from build123d import *

# Parameters (mm, degrees)
ESQUISSE1_W                   = 105
ESQUISSE1_H                   = 105
ESQUISSE1_W_2                 = 85
ESQUISSE1_H_2                 = 85
BOSS_EXTRU_3_DEPTH            = 88
BOSS_EXTRU_4_DEPTH            = 105
ESQUISSE7_W                   = 40
ESQUISSE7_H                   = 40
ESQUISSE7_W_2                 = 20
ESQUISSE7_H_2                 = 20
BOSS_EXTRU_11_DEPTH           = 110.5
ENL_V_MAT_EXTRU_9_REACH       = 242.562
ESQUISSE13_W                  = 10
ESQUISSE13_H                  = 20
BOSS_EXTRU_12_DEPTH           = 2.5
ESQUISSE17_R                  = 5
ESQUISSE17_W                  = 40
ESQUISSE17_H                  = 20
BOSS_EXTRU_13_DEPTH           = 52.5
ENL_V_MAT_EXTRU_12_DEPTH      = 265.326910813
ENL_V_MAT_EXTRU_12_DEPTH_BACK = 265.326910813
ESQUISSE18_R                  = 5
ENL_V_MAT_EXTRU_13_REACH      = 236.819
ESQUISSE19_W                  = 10
ESQUISSE19_H                  = 20
CONG_1_R                      = 10
ENL_V_MAT_EXTRU_15_DEPTH      = 88


with BuildPart() as part:
    # Esquisse1 → Boss.-Extru.3 (new body)
    with BuildSketch(Plane(origin=(0, 0, 0), x_dir=(1, 0, 0), z_dir=(0, 1, 0))):
        Rectangle(ESQUISSE1_W, ESQUISSE1_H)
        Rectangle(ESQUISSE1_W_2, ESQUISSE1_H_2, mode=Mode.SUBTRACT)
    extrude(amount=BOSS_EXTRU_3_DEPTH)

    # Esquisse3 → Boss.-Extru.4 (add)
    with BuildSketch(Plane.XY.offset(52.5)):
        Polygon((52.5, 6), (52.5, 0), (96.658434537, 0), (130.222419784, 40), (190.222419784, 40), (190.222419784, 46), (127.424573836, 46), (93.860588588, 6), align=None)
    extrude(amount=-BOSS_EXTRU_4_DEPTH)

    # Esquisse7 → Boss.-Extru.11 (add)
    with BuildSketch(Plane.XZ.offset(-40)):
        with Locations((190.222419784, 0)):
            Rectangle(ESQUISSE7_W, ESQUISSE7_H)
        with Locations((190.222419784, 0)):
            Rectangle(ESQUISSE7_W_2, ESQUISSE7_H_2, mode=Mode.SUBTRACT)
    extrude(amount=-BOSS_EXTRU_11_DEPTH)

    # Esquisse13 → Enlèv. mat.-Extru.9 (cut, up to next)
    with BuildSketch(Plane(origin=(0, 46, 0), x_dir=(1, 0, 0), z_dir=(0, 1, 0)), mode=Mode.PRIVATE) as enl_v_mat_extru_9_sk1:
        with Locations((185.222419784, 0)):
            Rectangle(ESQUISSE13_W, ESQUISSE13_H)
    enl_v_mat_extru_9_tool1 = extrude(enl_v_mat_extru_9_sk1.sketch, amount=-ENL_V_MAT_EXTRU_9_REACH, mode=Mode.PRIVATE) & part.part
    add(enl_v_mat_extru_9_tool1.solids().sort_by_distance((185.22242, 46, 0))[0], mode=Mode.SUBTRACT)

    # Esquisse14 → Boss.-Extru.12 (add, symmetric)
    with BuildSketch(Plane.XY):
        Polygon((52.5, 88), (101.965319391, 88), (154.40904634, 150.5), (170.222419784, 150.5), (170.222419784, 46), (127.424573836, 46), (93.860588588, 6), (52.5, 6), align=None)
    extrude(amount=BOSS_EXTRU_12_DEPTH, both=True)

    # Esquisse17 → Boss.-Extru.13 (add, symmetric)
    # profile 1 of 2: a face of its own
    with BuildSketch(Plane.XY):
        Polygon((44, 20), (44, 0), (77.5, 0), (77.5, 6), (77.5, 20), align=None)
        with Locations((67.5, 10)):
            Circle(ESQUISSE17_R, mode=Mode.SUBTRACT)
    # profile 2 of 2: a face of its own
    with BuildSketch(Plane.XY):
        with Locations((170.222419784, 50)):
            Rectangle(ESQUISSE17_W, ESQUISSE17_H)
        with Locations((160.222419784, 50)):
            Circle(ESQUISSE17_R, mode=Mode.SUBTRACT)
    extrude(amount=BOSS_EXTRU_13_DEPTH, both=True)

    # Esquisse18 → Enlèv. mat.-Extru.12 (cut, two sides: drawn at the far end of the back side and taken through both)
    with BuildSketch(Plane.XY.offset(2.5).offset(-ENL_V_MAT_EXTRU_12_DEPTH_BACK)):
        with Locations((160.222419784, 50)):
            Circle(ESQUISSE18_R)
        with Locations((67.5, 10)):
            Circle(ESQUISSE18_R)
    extrude(amount=ENL_V_MAT_EXTRU_12_DEPTH + ENL_V_MAT_EXTRU_12_DEPTH_BACK, mode=Mode.SUBTRACT)

    # Esquisse19 → Enlèv. mat.-Extru.13 (cut, up to next)
    with BuildSketch(Plane(origin=(0, 60, 0), x_dir=(1, 0, 0), z_dir=(0, 1, 0)), mode=Mode.PRIVATE) as enl_v_mat_extru_13_sk1:
        with Locations((185.222419784, 0)):
            Rectangle(ESQUISSE19_W, ESQUISSE19_H)
    enl_v_mat_extru_13_tool1 = extrude(enl_v_mat_extru_13_sk1.sketch, amount=-ENL_V_MAT_EXTRU_13_REACH, mode=Mode.PRIVATE) & part.part
    add(enl_v_mat_extru_13_tool1.solids().sort_by_distance((185.22242, 60, 0))[0], mode=Mode.SUBTRACT)

    # Congé1
    cong_1_edges = [part.edges().sort_by_distance(p)[0] for p in [
        (93.860588588, 6, 27.5),
        (127.424573836, 46, 27.5),
        (154.40904634, 150.5, 0),
        (101.965319391, 88, 0),
        (77.5, 20, 27.5),
        (77.5, 20, -27.5),
        (150.222419784, 60, 27.5),
        (150.222419784, 60, -27.5),
        (127.424573836, 46, -27.5),
        (93.860588588, 6, -27.5),
        (96.658434537, 0, 0),
        (130.222419784, 40, 0),
    ]]
    fillet(cong_1_edges, radius=CONG_1_R)

    # Esquisse20 → Enlèv. mat.-Extru.15 (cut)
    with BuildSketch(Plane(origin=(0, 0, 0), x_dir=(1, 0, 0), z_dir=(0, 1, 0))):
        Polygon((6, 52.5), (190.222419784, 20), (210.222419784, 20), (210.222419784, 52.5), align=None)
        Polygon((210.222419784, -20), (190.222419784, -20), (6, -52.5), (210.222419784, -52.5), align=None)
    extrude(amount=ENL_V_MAT_EXTRU_15_DEPTH, mode=Mode.SUBTRACT)


solid = part.part
Model file for the job. Use its own axes, mm. A direction names the side the tool comes from. Round coordinates to 2 decimals unless told otherwise and drop trailing zeros. Loops run counter-clockwise (first coordinate to the right, second up) from the corner with the lowest first, then second, coordinate; pieces in that order, holes last. Notation, with made-up numbers: (17.5, 55.25) -> (36.5, 55.25) arc R29 cw to (36.5, 79.25) -> close; hole circle Ø7 at (-21, 52.25). An arc over 180 degrees is marked (long way). Answer as CSV lines item,"result". Start each with the question number.
1) Slice it at A-A (y = 115.5). List the corners of the cut face in (x, z).
2) Probe line 1 along X through (y, z) = (50, 14); line 2 along Z through (x, y) = (183.5, 123.5); line 3 along X through (y, z) = (79, -20.5). List the from-to ranges inside material, lowest first.
3) Tool access for faces 4 (the face through (164, 40, 0)), 5 (the face through (180.222, 96, 0)), 6 (the face through (74.65, 16.99, -22.35)), 7 (the face through (52.5, 54, 24)): list every direction of +Z, -Z, +X, -X, +Y, -Y with a clear straight run to the whole face (end or side of a thin tool).
4) Slice it at B-B (y = 95). List the corners of the cut face in (x, z), plus the area to 3 significant figures.
5) Pin check, flat tips, straight feed: P1, Ø3.5, axis at x = 80.5, z = 20.5, coming from the +Y side; P2, Ø1, axis at x = 19, y = 24.5, coming from the +Z side; P3, Ø3, axis at y = 96, z = -22.5, coming from the -X side; P4, Ø13, axis at x = 160.22, y = 50, coming from the -Z side. Stop position of each tip, or through.
6) Mould opens along X. For faces 1 (the face through (49.92, 40.54, -44.75)), 2 (the face through (-52.5, 43, 1)), 3 (the face through (141, 46, 17)) say: +X half, -X half, draft (parallel to the pull), parting line (faces both ways), or undercut.
Filled in:
1,outline,"(125.04, -2.5) -> (170.22, -2.5) -> (170.22, -20) -> (210.22, -20) -> (210.22, 20) -> (170.22, 20) -> (170.22, 2.5) -> (125.04, 2.5) -> close; hole (180.22, -10) -> (200.22, -10) -> (200.22, 10) -> (180.22, 10) -> close"
2,line 1,"x = -52.5 to -42.5, 42.5 to 52.5, 150.22 to 155.22, 165.22 to 210.22"
2,line 2,"z = -20 to -10, 10 to 20"
2,line 3,"x = -52.5 to -42.5, 42.5 to 52.5"
3,face 4,"+Z, -Z, +X, -Y"
3,face 5,"+Y, -Y"
3,face 6,"-Z, +Y"
3,face 7,"+Z, +Y"
4,outline,"(107.84, -2.5) -> (170.22, -2.5) -> (170.22, -20) -> (210.22, -20) -> (210.22, 20) -> (170.22, 20) -> (170.22, 2.5) -> (107.84, 2.5) -> close; hole (180.22, -10) -> (200.22, -10) -> (200.22, 10) -> (180.22, 10) -> close"
4,area,"1,510 mm2"
5,P1,"stops at y = 6"
5,P2,"stops at z = 50.29"
5,P3,"passes through"
5,P4,"stops at z = -26.44"
6,face 1,"+X half"
6,face 2,"-X half"
6,face 3,"undercut"
